Design review of the part built by this model. Coordinates are the model's own, in mm. A direction names the side the tool comes from. Give positions to 0.01 mm unless a question says otherwise; leave off trailing zeros. Order: outer loops, then holes, each group sorted by start corner. A loop starts at its lowest first (then second) coordinate and runs counter-clockwise, first axis right, second up. Notation, with made-up numbers: M -38,65.25 L -2,65.25 A23 cw -2,91.25 Z; hole C 60.25,-33 d8. An arc over 180 degrees is marked long. Answer as a JSON object with one key per item and string values.
from build123d import *

# Parameters (mm, degrees)
F2_SIZE = 0.2
F3_W    = 0.65
F3_H    = 1
F5_R    = 0.2


with BuildPart() as f1:
    # F0 (on Front) → F1 (revolve)
    with BuildSketch(Plane.XZ):
        Polygon((0, -27), (0, 27), (-6, 27), (-6, 10), (-15, 10), (-15, -10), (-6, -10), (-6, -27), align=None)
    revolve(axis=Axis((0, 0, 3.962264), (0, 0, -1)))

    # F2
    f2_edges = [f1.edges().sort_by_distance(p)[0] for p in [
        (6, 0, 27),
        (15, 0, 10),
        (15, 0, -10),
        (6, 0, -27),
    ]]
    chamfer(f2_edges, length=F2_SIZE)

    # F3 (on Front) → F4 (revolve, cut)
    with BuildSketch(Plane.XZ):
        with Locations((-5.675, 25.7)):
            Rectangle(F3_W, F3_H)
        with Locations((-5.675, -25.7)):
            Rectangle(F3_W, F3_H)
    revolve(axis=Axis((0, 0, -1.776566), (0, 0, -1)), mode=Mode.SUBTRACT)

    # F5
    f5_edges = [f1.edges().sort_by_distance(p)[0] for p in [
        (6, 0, 10),
        (6, 0, -10),
    ]]
    fillet(f5_edges, radius=F5_R)


solid = f1.part
(1) We need section A-A (z = 5). Write out the cut boundary in (x, y), plus the area to 3 significant figures.
Checked values:
{"outline": "C 0,0 d30", "area": "707 mm^2"}
(2) To check wall thickness, follow L1, parallel to Z at x = -1.25, y = -8.5; L2, parallel to Y at x = 0, z = -17; L3, parallel to X at y = 9.25, z = 1. State the ranges of each line that lie inside material, in increasing order. Write a range as from..to.
Checked values:
{"L1": "z = -10..10", "L2": "y = -6..6", "L3": "x = -11.81..11.81"}
(3) Tool access review of faces 1 (the flat face through (0, 0, -27)), 2 (the cylindrical face through (14.985, 0.66, -0.137)), 3 (the flat face through (0.2, -6.4, -10)), 4 (the cylindrical face through (6, 0, 18)), 5 (the cylindrical face through (1.16, -5.223, -25.693)): name each direction out of +Z, -Z, +X, -X, +Y, -Y from which nothing blocks a thin tool from reaching the whole face with its end or side.
Checked values:
{"face 1": "-Z, +X, -X, +Y, -Y", "face 2": "+Z, -Z", "face 3": "-Z", "face 4": "+Z", "face 5": "none"}
(4) Insertion check: pin 1 (5 mm diameter, centred on x = -10.5, y = -8.5, fed in from -Z); pin 2 (10 mm diameter, centred on x = -12, z = 11, fed in from +Y); pin 3 (1.5 mm diameter, centred on x = 3, z = 21.5, fed in from -Y). Each pin has a flat end and moves straight along its axis. Give the tip position at first contact, or say it passes through.
Checked values:
{"pin 1": "stops at z = -10", "pin 2": "stops at y = 13.19", "pin 3": "stops at y = -5.56"}
(5) We need section B-B (z = 17). Write out the cut boundary in (x, y), plus the area to 3 significant figures.
Checked values:
{"outline": "C 0,0 d12", "area": "113 mm^2"}
